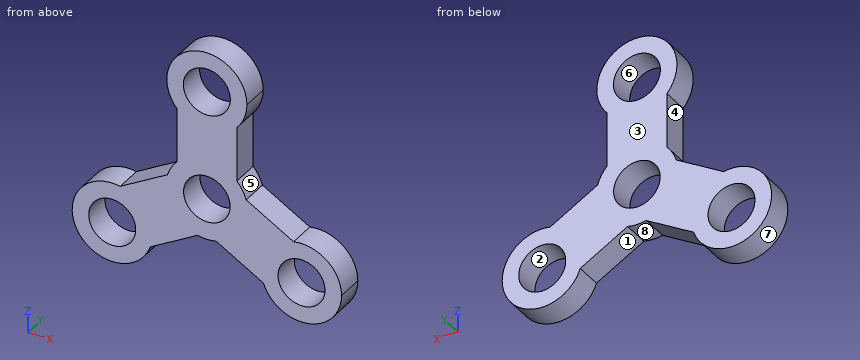
```python
from build123d import *

# Parameters (mm, degrees)
F0_R     = 10.890936
F0_R_2   = 10.799032
F1_DEPTH = 12.7


with BuildPart() as f1:
    # F0 (on Front) → F1 (new body)
    with BuildSketch(Plane.XZ):
        with BuildLine():
            ThreePointArc((13.928364, 38.366641), (17.3715, 44.084221), (18.57085, 50.649848))
            ThreePointArc((18.57085, 50.649848), (-6.565627, 68.021348), (-13.928364, 38.366641))
            ThreePointArc((-13.928364, 38.366641), (0, 32.078998), (13.928364, 38.366641))
        make_face()
        with Locations((0, 50.649848)):
            Circle(F0_R, mode=Mode.SUBTRACT)
        with BuildLine():
            ThreePointArc((13.928364, 38.366641), (0, 32.078998), (-13.928364, 38.366641))
            Line((-13.928364, 38.366641), (-13.928364, 13.030285))
            ThreePointArc((-13.928364, 13.030285), (0, 19.073218), (13.928364, 13.030285))
            Line((13.928364, 13.030285), (13.928364, 38.366641))
        make_face()
        with BuildLine():
            ThreePointArc((-4.320376, -18.577459), (-16.517891, -9.536609), (-18.248739, 5.547174))
            Line((-18.248739, 5.547174), (-40.190668, -7.121004))
            ThreePointArc((-40.190668, -7.121004), (-29.492305, -13.563577), (-25.293205, -25.324924))
            ThreePointArc((-25.293205, -25.324924), (-25.537081, -28.324674), (-26.262304, -31.245637))
            Line((-26.262304, -31.245637), (-4.320376, -18.577459))
        make_face()
        with BuildLine():
            ThreePointArc((13.928364, 13.030285), (0, 19.073218), (-13.928364, 13.030285))
            ThreePointArc((-13.928364, 13.030285), (-16.517891, 9.536609), (-18.248739, 5.547174))
            ThreePointArc((-18.248739, 5.547174), (-16.517891, -9.536609), (-4.320376, -18.577459))
            ThreePointArc((-4.320376, -18.577459), (0, -19.073218), (4.320376, -18.577459))
            ThreePointArc((4.320376, -18.577459), (14.936383, -11.861369), (19.073218, 0))
            ThreePointArc((19.073218, 0), (18.865972, 2.804055), (18.248739, 5.547174))
            ThreePointArc((18.248739, 5.547174), (16.517891, 9.536609), (13.928364, 13.030285))
        make_face()
        Circle(F0_R_2, mode=Mode.SUBTRACT)
        with BuildLine():
            ThreePointArc((-25.293205, -25.324924), (-29.492305, -13.563577), (-40.190668, -7.121004))
            ThreePointArc((-40.190668, -7.121004), (-59.946883, -34.610349), (-26.262304, -31.245637))
            ThreePointArc((-26.262304, -31.245637), (-25.537081, -28.324674), (-25.293205, -25.324924))
        make_face()
        with Locations((-43.864055, -25.324924)):
            Circle(F0_R, mode=Mode.SUBTRACT)
        with BuildLine():
            Line((40.190668, -7.121004), (18.248739, 5.547174))
            ThreePointArc((18.248739, 5.547174), (18.865972, 2.804055), (19.073218, 0))
            ThreePointArc((19.073218, 0), (14.936383, -11.861369), (4.320376, -18.577459))
            Line((4.320376, -18.577459), (26.262304, -31.245637))
            ThreePointArc((26.262304, -31.245637), (27.781227, -16.039499), (40.190668, -7.121004))
        make_face()
        with BuildLine():
            ThreePointArc((62.434905, -25.324924), (55.625402, -10.953174), (40.190668, -7.121004))
            ThreePointArc((40.190668, -7.121004), (27.781227, -16.039499), (26.262304, -31.245637))
            ThreePointArc((26.262304, -31.245637), (46.863805, -43.651898), (62.434905, -25.324924))
        make_face()
        with Locations((43.864055, -25.324924)):
            Circle(F0_R, mode=Mode.SUBTRACT)
    extrude(amount=F1_DEPTH)


solid = f1.part
```
Work out the finished part from the listing and answer in its coordinate system (mm). Face numbers are marked on the shaded views. A direction names the side the tool comes from. Give positions to 0.01 mm unless a question says otherwise; leave off trailing zeros. Write each loop counter-clockwise with the first axis right and the second up, starting at its lowest first coordinate (ties: lowest second). Pieces come first, ordered by that corner, then holes. Notation, with made-up numbers: (-27, 18.5) - (16, 18.5) arc R17 cw to (16, 47.5) - close; hole circle Ø3 at (82.25, -13.75). An arc over 180 degrees is marked (long way). Use one line per item in the form item = value.
1. A cutting plane is placed at B-B (x = 0). Write down the section's boundary in (y, z).
Filled in:
outline = (-12.7, -19.07) - (0, -19.07) - (0, -10.8) - (-12.7, -10.8) - close; (-12.7, 10.8) - (0, 10.8) - (0, 39.76) - (-12.7, 39.76) - close; (-12.7, 61.54) - (0, 61.54) - (0, 69.22) - (-12.7, 69.22) - close
2. A cutting plane is placed at D-D (x = -42). Write down the section's boundary in (y, z), and give its area (3 significant figures).
Filled in:
outline = (-12.7, -43.8) - (0, -43.8) - (0, -36.06) - (-12.7, -36.06) - close; (-12.7, -14.59) - (0, -14.59) - (0, -6.85) - (-12.7, -6.85) - close
area = 197 mm^2
3. For the marked faces 1, 2, 3, 4 and 5, determine the directions among +Z, -Z, +X, -X, +Y, -Y from which every point of the face is accessible in a straight line to the end or side of a thin tool.
Filled in:
face_1 = -Z, +Y, -Y
face_2 = +Y, -Y
face_3 = +Z, -Z, +X, -X, +Y
face_4 = -X, +Y, -Y
face_5 = +X, +Y, -Y
4. A cutting plane is placed at A-A (y = -9). Write down the section's boundary in (x, z) (3 decimals), and give its area (3 significant figures).
Filled in:
outline = (-40.191, -7.121) arc R18.571 ccw (long way) to (-26.262, -31.246) - (-4.32, -18.577) arc R19.073 ccw to (4.32, -18.577) - (26.262, -31.246) arc R18.571 ccw (long way) to (40.191, -7.121) - (18.249, 5.547) arc R19.073 ccw to (13.928, 13.03) - (13.928, 38.367) arc R18.571 ccw to (18.571, 50.65) arc R18.571 ccw (long way) to (-13.928, 38.367) - (-13.928, 13.03) arc R19.073 ccw to (-18.249, 5.547) - close; hole circle Ø21.782 at (-43.864, -25.325); hole circle Ø21.782 at (0, 50.65); hole circle Ø21.598 at (0, 0); hole circle Ø21.782 at (43.864, -25.325)
area = 4,310 mm^2
5. A cutting plane is placed at C-C (z = 59). Write down the section's boundary in (x, y), and give its area (3 significant figures).
Filled in:
outline = (-16.59, -12.7) - (-6.99, -12.7) - (-6.99, 0) - (-16.59, 0) - close; (6.99, -12.7) - (16.59, -12.7) - (16.59, 0) - (6.99, 0) - close
area = 244 mm^2
6. Each of these flat-tipped pins is pushed along its axis until it touches: pin 1 Ø2 at (y, z) = (-6, 40) entering from -X; pin 2 Ø4 at (y, z) = (-5, 15) entering from +X; pin 3 Ø8 at (x, z) = (-12.5, 2.5) entering from +Y; pin 4 Ø2 at (y, z) = (-8.5, 48.5) entering from -X. Where does it stop, or does it pass through?
Filled in:
pin_1 = -15.87
pin_2 = 13.96
pin_3 = 0
pin_4 = -18.54
7. Consider L1, parallel to X at y = -0.5, z = -27.5; L2, parallel to Z at x = -8, y = -12; L3, parallel to X at y = -7.75, z = 31. Determine where each line is inside the solid, lowest interval first.
Filled in:
L1 = -62.31 to -54.54, -33.19 to -19.77, 19.77 to 33.19, 54.54 to 62.31
L2 = -20.7 to -7.25, 7.25 to 43.26, 58.04 to 67.41
L3 = -13.93 to 13.93
8. Determine the mould class of the marked faces 6, 7 and 8 for opening direction Z: released by +Z, released by -Z, zero draft, split by the parting line, or undercut.
Filled in:
face_6 = undercut
face_7 = split by the parting line
face_8 = released by -Z
